Job drawing, mm, ordinate dimensions from the low corner. One solid piece. A direction names the side the tool comes from. Give positions to 0.01 mm unless a question says otherwise; leave off trailing zeros. Loops run counter-clockwise (first coordinate to the right, second up) from the corner with the lowest first, then second, coordinate; pieces in that order, holes last. Notation, with made-up numbers: (2.25, 13) -> (36.25, 13) arc R11 cw to (36.25, 19) -> close; hole circle Ø8 at (37.5, -32). An arc over 180 degrees is marked (long way). Answer as a JSON object with one key per item and string values. Group by question number.
Q1. Tool access for the marked faces 5 and 6: list every direction of +Z, -Z, +X, -X, +Y, -Y with a clear straight run to the whole face (end or side of a thin tool).
Q2. Band-saw the part on D-D, the plane y = 146.5. Write the cut outline in (x, z), plus the area to 3 significant figures.
Q3. Band-saw the part on A-A, the plane z = 80. Write the cut outline in (x, y).
Q4. Wall check: probe 1 along Z at (x, y) = (100, 20.5) (1 decimal); probe 2 along Z at (x, y) = (95, 33.5); probe 3 along X at (y, z) = (46, 101.5). Give the ranges that are in metal, low to high. Write a range as from..to.
Q5. Drop flat-ended pins along their axis: pin 1 (2 mm diameter, centred on x = 69, z = 81.5, fed in from +Y); pin 2 (1.5 mm diameter, centred on x = 109.5, z = 128.5, fed in from -Y); pin 3 (5 mm diameter, centred on x = 101.5, z = 90.5, fed in from -Y); pin 4 (1 mm diameter, centred on x = 97, z = 29, fed in from +Y). Give the stop position or say it passes through.
Q6. Two-plate mould, pull along X, no slides. Class the marked faces 1, 2, 3 and 4: pulls with the +X half, pulls with the -X half, needs draft (parallel to the pull), parting line crosses it, or undercut.
Q7. Band-saw the part on B-B, the plane x = 100. Write the cut outline in (y, z) (1 decimal).
Q8. Band-saw the part on C-C, the plane z = 143.5. Write the cut outline in (x, y).
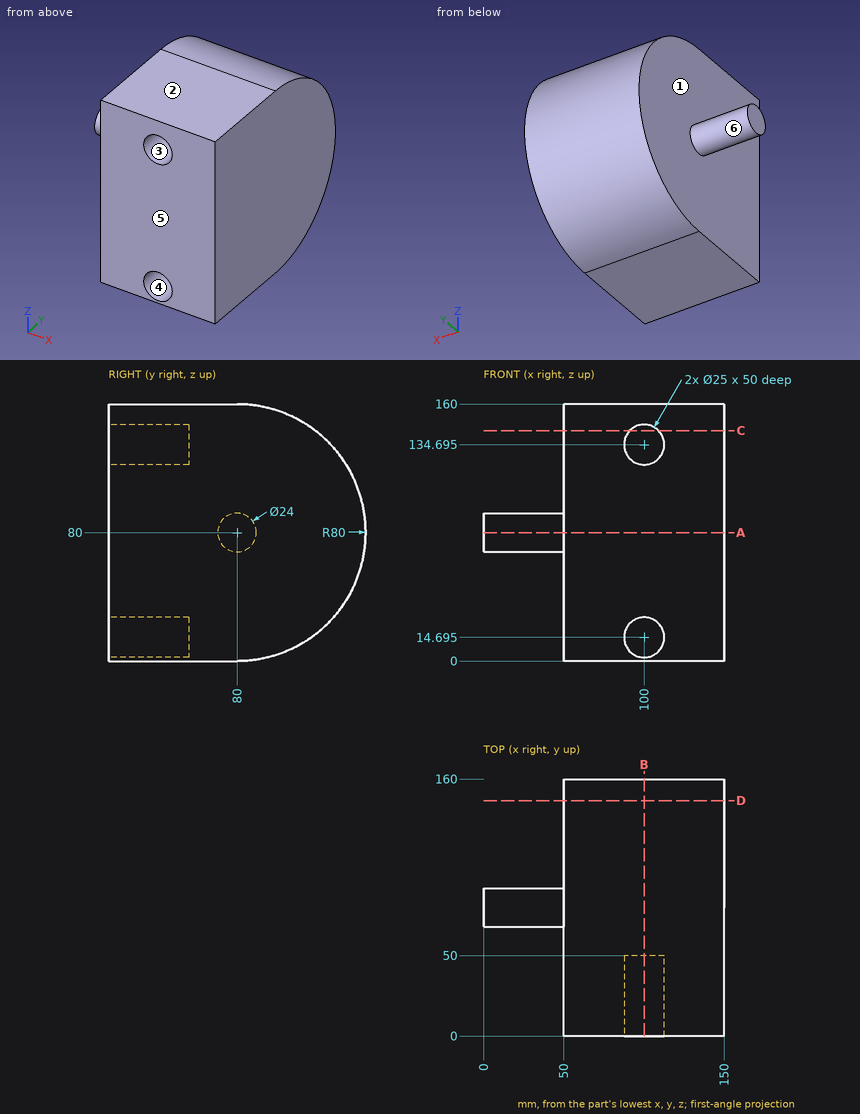
Worked answers:
{
 "1": {"face 5": "+Z, -Z, +X, -X, -Y", "face 6": "-X"},
 "2": {"outline": "(50, 35.53) -> (150, 35.53) -> (150, 124.47) -> (50, 124.47) -> close", "area": "8,890 mm2"},
 "3": {"outline": "(0, 68) -> (50, 68) -> (50, 0) -> (150, 0) -> (150, 160) -> (50, 160) -> (50, 92) -> (0, 92) -> close"},
 "4": {"probe 1": "0..2.2, 27.2..122.2, 147.2..160", "probe 2": "0..3.24, 26.15..123.24, 146.15..160", "probe 3": "50..150"},
 "5": {"pin 1": "y = 160", "pin 2": "y = 50", "pin 3": "y = 0", "pin 4": "y = 142.05"},
 "6": {"face 1": "pulls with the -X half", "face 2": "needs draft", "face 3": "undercut", "face 4": "undercut"},
 "7": {"outline": "(0, 0) -> (80, 0) arc R80 ccw to (80, 160) -> (0, 160) -> (0, 147.2) -> (50, 147.2) -> (50, 122.2) -> (0, 122.2) -> (0, 27.2) -> (50, 27.2) -> (50, 2.2) -> (0, 2.2) -> close"},
 "8": {"outline": "(50, 0) -> (91.13, 0) -> (91.13, 50) -> (108.87, 50) -> (108.87, 0) -> (150, 0) -> (150, 128.66) -> (50, 128.66) -> close"}
}
